For this review, take the finished solid that the model builds, in its own axes (mm). Give positions to 0.01 mm unless a question says otherwise; leave off trailing zeros. Write each loop counter-clockwise with the first axis right and the second up, starting at its lowest first coordinate (ties: lowest second). Pieces come first, ordered by that corner, then holes.
1) We need section D-D on y = 44.5. Give the boundary of the cut face in (x, z), and give its area (3 significant figures).
2) For P1, Ø0.6, axis at y = 48.5, z = 1, coming from the +X side; P2, Ø1, axis at x = -50, z = 0.5, coming from the -Y side; P3, Ø2.5, axis at x = -15, y = -15, coming from the +Z side; P4, Ø0.6, axis at x = -51.5, z = 0.5, coming from the +Y side, all flat-tipped, find the tip position at first contact; note any pin that passes through.
3) We need section A-A on x = -15. Give the boundary of the cut face in (y, z), and give its area (3 significant figures).
4) Wall thickness on line 1 along Y through (x, z) = (-15, 1.1); line 2 along Y through (x, z) = (-16, 1.5): over which ranges is each line inside the solid? List them lowest first.
5) We need section C-C on z = 1.65. Give the boundary of the cut face in (x, y), and give its area (3 significant figures).
6) Draft analysis for pull direction Y (two halves, no side actions). For faces 1 (the face through (-1, 1, 2)), 2 (the face through (16.5, 14.93, 1.01)), state which applies: pulls with the +Y half, pulls with the -Y half, needs draft (parallel to the pull), parting line crosses it, or undercut.
from build123d import *

# Parameters (mm, degrees)
F2_DEPTH = 2
F3_D     = 3


with BuildPart() as f2:
    # F0 (on Top) → F2 (new body)
    with BuildSketch(Plane.XY):
        Polygon((40, 60), (0, 60), (-4.426457, 60), (-40, 60), (-40, 40), (-60, 40), (-60, 0), (-60, -40), (-40, -40), (-40, -60), (0, -60), (40, -60), (40, -40), (60, -40), (60, 0), (60, 40), (40, 40), align=None)
    extrude(amount=F2_DEPTH)

    # F3 (through all)
    with Locations(Plane(origin=(0, 0, 0), x_dir=(1, 0, 0), z_dir=(0, 0, -1))):
        with Locations((-15, 15), (15, 15), (-15, -15), (15, -15)):
            Hole(F3_D / 2)


solid = f2.part
Results list:
1. outline: (-40, 0) - (40, 0) - (40, 2) - (-40, 2) - close
1. area: 160 mm2
2. P1: stops at x = 40
2. P2: stops at y = -40
2. P3: passes through
2. P4: stops at y = 40
3. outline: (-60, 0) - (-16.5, 0) - (-16.5, 2) - (-60, 2) - close; (-13.5, 0) - (13.5, 0) - (13.5, 2) - (-13.5, 2) - close; (16.5, 0) - (60, 0) - (60, 2) - (16.5, 2) - close
3. area: 228 mm2
4. line 1: y = -60 to -16.5, -13.5 to 13.5, 16.5 to 60
4. line 2: y = -60 to -16.12, -13.88 to 13.88, 16.12 to 60
5. outline: (-60, -40) - (-40, -40) - (-40, -60) - (40, -60) - (40, -40) - (60, -40) - (60, 40) - (40, 40) - (40, 60) - (-40, 60) - (-40, 40) - (-60, 40) - close; hole circle Ø3 at (-15, -15); hole circle Ø3 at (-15, 15); hole circle Ø3 at (15, -15); hole circle Ø3 at (15, 15)
5. area: 12,800 mm2
6. face 1: needs draft
6. face 2: undercut
